Source: CAD feature listing. Evaluate the final solid. Frame: model axes, mm. Face numbers are marked on the shaded views. A direction names the side the tool comes from. Round coordinates to 2 decimals unless told otherwise and drop trailing zeros. Write each loop counter-clockwise with the first axis right and the second up, starting at its lowest first coordinate (ties: lowest second). Pieces come first, ordered by that corner, then holes.
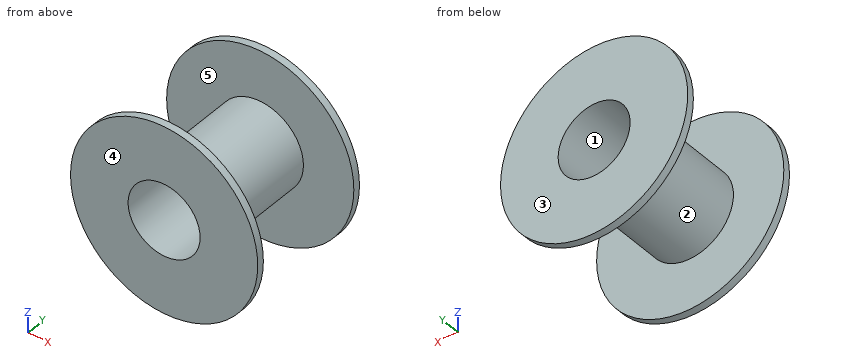
from build123d import *

# Parameters (mm, degrees)
F0_R     = 6.5
F0_R_2   = 2.5
F1_DEPTH = 0.5
F2_R     = 3
F2_R_2   = 2.5
F3_DEPTH = 8
F4_R     = 6.5
F4_R_2   = 2.5
F5_DEPTH = 0.5
F7_R     = 6.5
F7_R_2   = 2.5
F8_DEPTH = 0.5


with BuildPart() as f1:
    # F0 (on Front) → F1 (new body)
    with BuildSketch(Plane.XZ):
        Circle(F0_R)
        Circle(F0_R_2, mode=Mode.SUBTRACT)
    extrude(amount=F1_DEPTH)

    # F2 (on face) → F3 (join)
    with BuildSketch(Plane.XZ.offset(0.5)):
        Circle(F2_R)
        Circle(F2_R_2, mode=Mode.SUBTRACT)
    extrude(amount=F3_DEPTH)

    # F7 (on face) → F8 (join)
    with BuildSketch(Plane.XZ.offset(8.5)):
        Circle(F7_R)
        Circle(F7_R_2, mode=Mode.SUBTRACT)
    extrude(amount=F8_DEPTH)


with BuildPart() as f5:
    # F4 (on face) → F5 (new body)
    with BuildSketch(Plane.XZ):
        Circle(F4_R)
        Circle(F4_R_2, mode=Mode.SUBTRACT)
    extrude(amount=F5_DEPTH)


solid = f1.part
1) Contact query for flat-ended pins moving along their axis: P1, Ø6.5, axis at x = 0, z = 0, coming from the -Y side; P2, Ø1, axis at y = -7.5, z = 2.5, coming from the +X side; P3, Ø3, axis at x = 3.5, y = -6.5, coming from the +Z side. Output: stop coordinate, or through.
Taken from the geometry:
P1: stops at y = -9
P2: stops at x = 2.24
P3: stops at z = 2.24
2) Section query A-A on z = 0. Return the cut outline in (x, y).
Taken from the geometry:
outline: (-6.5, -9) - (-2.5, -9) - (-2.5, 0) - (-6.5, 0) - (-6.5, -0.5) - (-3, -0.5) - (-3, -8.5) - (-6.5, -8.5) - close; (2.5, -9) - (6.5, -9) - (6.5, -8.5) - (3, -8.5) - (3, -0.5) - (6.5, -0.5) - (6.5, 0) - (2.5, 0) - close
3) Section query D-D on x = -4.5. Return the cut outline in (y, z), then the cut area to 3 significant figures.
Taken from the geometry:
outline: (-9, -4.69) - (-8.5, -4.69) - (-8.5, 4.69) - (-9, 4.69) - close; (-0.5, -4.69) - (0, -4.69) - (0, 4.69) - (-0.5, 4.69) - close
area: 9.38 mm2
4) Material intervals for line 1 (Y direction, x = -3.75, z = -2.5); line 2 (Z direction, x = 0, y = -2.5); line 3 (X direction, y = -5, z = -1), sorted ascending.
Taken from the geometry:
line 1: y = -9 to -8.5, -0.5 to 0
line 2: z = -3 to -2.5, 2.5 to 3
line 3: x = -2.83 to -2.29, 2.29 to 2.83
5) Section query C-C on y = -6.5. Return the cut outline in (x, z).
Taken from the geometry:
outline: circle Ø6 at (0, 0); hole circle Ø5 at (0, 0)
6) Section query B-B on x = 0. Return the cut outline in (y, z).
Taken from the geometry:
outline: (-9, -6.5) - (-8.5, -6.5) - (-8.5, -3) - (-0.5, -3) - (-0.5, -6.5) - (0, -6.5) - (0, -2.5) - (-9, -2.5) - close; (-9, 2.5) - (0, 2.5) - (0, 6.5) - (-0.5, 6.5) - (-0.5, 3) - (-8.5, 3) - (-8.5, 6.5) - (-9, 6.5) - close
7) Pull-direction query (Y, two-part tool) for the marked faces 3, 4 and 5; classes: released by +Y, released by -Y, zero draft, split by the parting line, or undercut.
Taken from the geometry:
face 3: released by +Y
face 4: released by -Y
face 5: undercut
8) Reachability of the marked faces 1 and 2 from +Z, -Z, +X, -X, +Y, -Y: full face, straight path, thin tool, end or side. Return the list, or none.
Taken from the geometry:
face 1: +Y, -Y
face 2: none
